```python
from build123d import *

# Parameters (mm, degrees)
SKETCH_1_R               = 3
EXTRUDE_1_DEPTH          = 10
M3X0_5_1_D               = 2.5
M3X0_5_1_DEPTH           = 6.5
M3X0_5_1_TIP             = 0.751075774
M3X0_5_1_ON_FACE_2_D     = 2.5
M3X0_5_1_ON_FACE_2_DEPTH = 6.5
M3X0_5_1_ON_FACE_2_TIP   = 0.751075774
SKETCH_3_R               = 1.25
CUT_EXTRUDE_1_DEPTH      = 20


with BuildPart() as part:
    # ｽｹｯﾁ1 → ﾎﾞｽ - 押し出し1 (new body, symmetric)
    with BuildSketch(Plane.XY):
        Circle(SKETCH_1_R)
    extrude(amount=EXTRUDE_1_DEPTH, both=True)

    # M3x0.5 ねじ穴1
    with Locations(Plane.XY.offset(10)):
        with Locations((0, 0)):
            Hole(M3X0_5_1_D / 2, depth=M3X0_5_1_DEPTH)
            with Locations((0, 0, -(M3X0_5_1_DEPTH + M3X0_5_1_TIP / 2))):  # 118° drill point
                Cone(0, M3X0_5_1_D / 2, M3X0_5_1_TIP, mode=Mode.SUBTRACT)

    # M3x0.5 ねじ穴1 on face 2
    with Locations(Plane(origin=(0, 0, -10), x_dir=(-1, 0, 0), z_dir=(0, 0, -1))):
        with Locations((0, 0)):
            Hole(M3X0_5_1_ON_FACE_2_D / 2, depth=M3X0_5_1_ON_FACE_2_DEPTH)
            with Locations((0, 0, -(M3X0_5_1_ON_FACE_2_DEPTH + M3X0_5_1_ON_FACE_2_TIP / 2))):  # 118° drill point
                Cone(0, M3X0_5_1_ON_FACE_2_D / 2, M3X0_5_1_ON_FACE_2_TIP, mode=Mode.SUBTRACT)

    # ｽｹｯﾁ3 → ｶｯﾄ - 押し出し1 (cut)
    with BuildSketch(Plane(origin=(0, 0, -10), x_dir=(-1, 0, 0), z_dir=(0, 0, -1))):
        Circle(SKETCH_3_R)
    extrude(amount=-CUT_EXTRUDE_1_DEPTH, mode=Mode.SUBTRACT)


solid = part.part
```
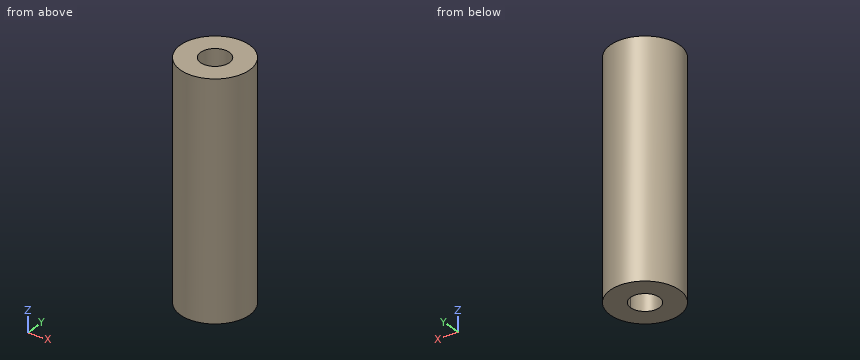
Part model, mm, in its own coordinate system. Coordinates: 2 decimals unless noted, no trailing zeros. Order: outer loops, then holes, each group sorted by start corner. A loop starts at its lowest first (then second) coordinate and runs counter-clockwise, first axis right, second up. Notation, with made-up numbers: (34, -24.5) -> (47, -24.5) arc R21 cw to (47, -13.5) -> close; hole circle Ø2 at (19.25, 26). An arc over 180 degrees is marked (long way). Put each result on its own line as item: value. Start each with the question number.
(1) Band-saw the part on A-A (x = 0). Give the cut face in (y, z), then the cut area to 3 significant figures.
(2) Probe line 1 along Y through (x, z) = (0, 8); line 2 along Y through (x, z) = (-1.1, 8.5); line 3 along Y through (x, z) = (-1.5, -4.5). List the from-to ranges inside material, lowest first. Write a range as [from, to].
(3) Band-saw the part on D-D (y = -1.8). Give the cut face in (x, z), then the cut area to 3 significant figures.
(4) Band-saw the part on B-B (y = -0.95). Give the cut face in (x, z).
(5) Band-saw the part on C-C (z = -5.5). Give the cut face in (x, y).
(6) Pin check, flat tips, straight feed: pin 1 Ø3 at (y, z) = (1.5, 7) entering from -X; pin 2 Ø1.5 at (x, y) = (0, 0) entering from +Z; pin 3 Ø1 at (x, z) = (2, 5.5) entering from +Y; pin 4 Ø1.5 at (x, z) = (1, 6.5) entering from +Y. Stop position of each tip, or through.
Determined:
1. outline: (-3, -10) -> (-1.25, -10) -> (-1.25, 10) -> (-3, 10) -> close; (1.25, -10) -> (3, -10) -> (3, 10) -> (1.25, 10) -> close
1. area: 70.0 mm²
2. line 1: y = [-3, -1.25], [1.25, 3]
2. line 2: y = [-2.79, -0.59], [0.59, 2.79]
2. line 3: y = [-2.6, 2.6]
3. outline: (-2.4, -10) -> (2.4, -10) -> (2.4, 10) -> (-2.4, 10) -> close
3. area: 96.0 mm²
4. outline: (-2.85, -10) -> (-0.81, -10) -> (-0.81, 10) -> (-2.85, 10) -> close; (0.81, -10) -> (2.85, -10) -> (2.85, 10) -> (0.81, 10) -> close
5. outline: circle Ø6 at (0, 0); hole circle Ø2.5 at (0, 0)
6. pin 1: stops at x = -3
6. pin 2: passes through
6. pin 3: stops at y = 2.6
6. pin 4: stops at y = 2.99
